CAD build for the part. Positions are in the model's coordinates, mm. Face numbers are marked on the shaded views. A direction names the side the tool comes from. Give positions to 0.01 mm unless a question says otherwise; leave off trailing zeros. Loops run counter-clockwise (first coordinate to the right, second up) from the corner with the lowest first, then second, coordinate; pieces in that order, holes last. Notation, with made-up numbers: M 45,-30 L 97,-30 A31 cw 97,-6 Z; hole C -19,75.5 d8. An arc over 180 degrees is marked long. One line per question, with ' | ' between items.
```python
from build123d import *

# Parameters (mm, degrees)
SKETCH_1_W      = 20
SKETCH_1_H      = 6
SKETCH_1_R      = 1.4
EXTRUDE_1_DEPTH = 3
SKETCH_2_W      = 20
SKETCH_2_H      = 15
EXTRUDE_2_DEPTH = 2.5
EXTRUDE_3_DEPTH = 20
CHAMFER_1_SIZE  = 1.2


with BuildPart() as part:
    # 草图1 → 凸台-拉伸1 (new body)
    with BuildSketch(Plane(origin=(0, 0, 0), x_dir=(1, 0, 0), z_dir=(0, 1, 0))):
        Rectangle(SKETCH_1_W, SKETCH_1_H)
        with Locations((-7, 0)):
            Circle(SKETCH_1_R, mode=Mode.SUBTRACT)
        with Locations((7, 0)):
            Circle(SKETCH_1_R, mode=Mode.SUBTRACT)
    extrude(amount=EXTRUDE_1_DEPTH)

    # 草图2 → 凸台-拉伸2 (add)
    with BuildSketch(Plane(origin=(0, 3, 0), x_dir=(1, 0, 0), z_dir=(0, 1, 0))):
        with Locations((0, -4.5)):
            Rectangle(SKETCH_2_W, SKETCH_2_H)
    extrude(amount=EXTRUDE_2_DEPTH)

    # 草图3 → 凸台-拉伸3 (add)
    with BuildSketch(Plane.ZY.offset(10)):
        Polygon((-3, 5.5), (-8.5, 0), (-3, 0), align=None)
    extrude(amount=-EXTRUDE_3_DEPTH)

    # 倒角1
    chamfer_1_edges = [part.edges().sort_by_distance(p)[0] for p in [
        (0, 3, 3),
        (-10, 3, 7.5),
        (0, 3, 12),
        (10, 3, 7.5),
        (-10, 5.5, 4.5),
        (0, 5.5, 12),
        (10, 5.5, 4.5),
        (10, 2.75, -5.75),
        (-10, 2.75, -5.75),
        (10, 1.5, 3),
        (-10, 1.5, 3),
    ]]
    chamfer(chamfer_1_edges, length=CHAMFER_1_SIZE)


solid = part.part
```
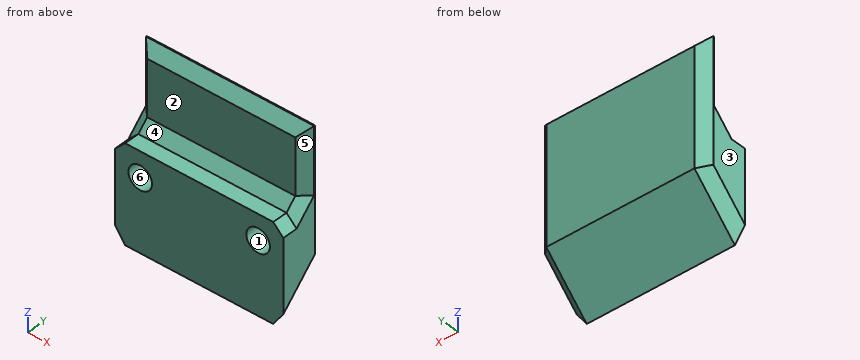
Item 1: Saw through at C-C on y = 1.05. Give the cut face in (x, z), and give its area (3 significant figures).
Conclusion:
outline: M -10,-5.75 L -8.8,-7.45 L 8.8,-7.45 L 10,-5.75 L 10,1.8 L 8.8,3 L -8.8,3 L -10,1.8 Z; hole C -7,0 d2.8; hole C 7,0 d2.8 | area: 193 mm²
Item 2: Drop flat-ended pins along their axis: P1, Ø0.8, axis at x = 7, z = 0, coming from the -Y side; P2, Ø0.5, axis at x = -0.5, y = 1, coming from the +Z side; P3, Ø5.5, axis at x = 3.5, z = 6.5, coming from the -Y side. Give the stop position or say it passes through.
Conclusion:
P1: y = 3 | P2: z = 3 | P3: y = 2.55
Item 3: Saw through at A-A on z = 2.5. Give the cut face in (x, y), and give its area (3 significant figures).
Conclusion:
outline: M -10,2.5 L -9.3,1.8 L -9.3,0 L 9.3,0 L 9.3,1.8 L 10,2.5 L 10,4.3 L 8.8,5.5 L -8.8,5.5 L -10,4.3 Z | area: 106 mm²
Item 4: Drill centre lines: line 1 along X through (y, z) = (2, 0); line 2 along Y through (x, z) = (1.75, -5.5); line 3 along Z through (x, y) = (-7, 1.15). Where is each one in solid material? Low to high. Write a range as [from, to].
Conclusion:
line 1: [-10, -8.4], [-5.6, 5.6], [8.4, 10] | line 2: [0, 3] | line 3: [-7.35, -1.4], [1.4, 3]
Item 5: Mould opens along X. For the marked faces 1, 2 and 3 say: pulls with the +X half, pulls with the -X half, needs draft (parallel to the pull), parting line crosses it, or undercut.
Conclusion:
face 1: undercut | face 2: needs draft | face 3: pulls with the -X half
Item 6: Saw through at B-B on x = -2.5. Give the cut face in (y, z), and give its area (3 significant figures).
Conclusion:
outline: M 0,-8.5 L 5.5,-3 L 5.5,10.8 L 4.3,12 L 4.2,12 L 3,10.8 L 3,4.2 L 1.8,3 L 0,3 Z | area: 69.9 mm²
Item 7: Saw through at D-D on z = 0. Give the cut face in (x, y).
Conclusion:
outline: M -10,0 L -8.4,0 L -8.4,3 L -5.6,3 L -5.6,0 L 5.6,0 L 5.6,3 L 8.4,3 L 8.4,0 L 10,0 L 10,4.3 L 8.8,5.5 L -8.8,5.5 L -10,4.3 Z
Item 8: 3-axis set-ups, long thin cutter, end or side, ignore diameter. For the marked faces 4, 5 and 6: which of +Z, -Z, +X, -X, +Y, -Y reach the whole face in a straight line?
Conclusion:
face 4: +Z, +X, -X, -Y | face 5: +Z, +X, -Y | face 6: -Y
